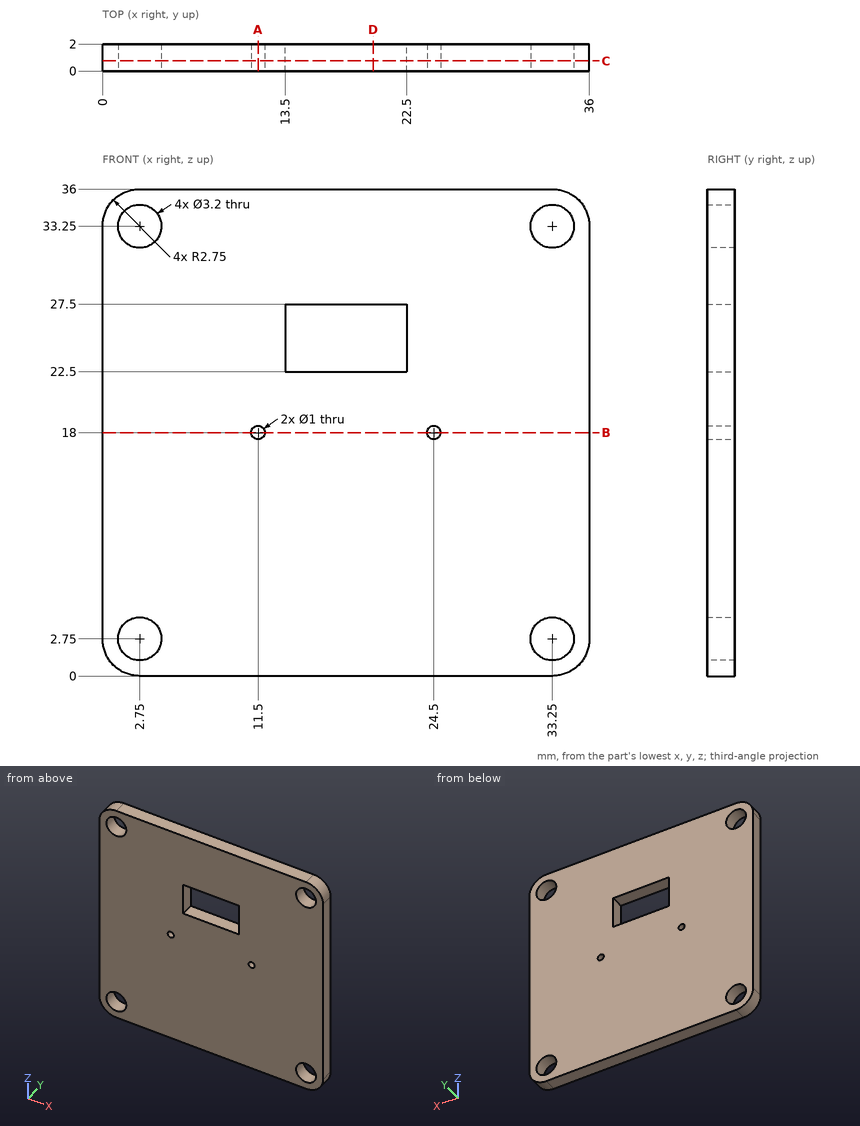
The drawing under review shows one solid part. Ordinate dimensions are in mm from its lowest x, y, z. Round coordinates to 2 decimals unless told otherwise and drop trailing zeros. Order: outer loops, then holes, each group sorted by start corner. A loop starts at its lowest first (then second) coordinate and runs counter-clockwise, first axis right, second up. Notation, with made-up numbers: (7.25, 78) -> (24.25, 78) arc R11 ccw to (24.25, 83) -> close; hole circle Ø8 at (48.5, 10.5). An arc over 180 degrees is marked (long way). Return JSON: item names as keys, results as strings.
1. For L1, parallel to X at y = 0.9, z = 33.25; L2, parallel to X at y = 1.15, z = 18; L3, parallel to Z at x = 16.5, y = 0.6, list the stretches that pass through material, from the lowest coordinate up. Write a range as [from, to].
Answer block:
{"L1": "x = [0, 1.15], [4.35, 31.65], [34.85, 36]", "L2": "x = [0, 11], [12, 24], [25, 36]", "L3": "z = [0, 22.5], [27.5, 36]"}
2. Take a section at B-B (z = 18). Write out the cut boundary in (x, y), then the cut area to 3 significant figures.
Answer block:
{"outline": "(0, 0) -> (11, 0) -> (11, 2) -> (0, 2) -> close; (12, 0) -> (24, 0) -> (24, 2) -> (12, 2) -> close; (25, 0) -> (36, 0) -> (36, 2) -> (25, 2) -> close", "area": "68.0 mm²"}
3. Take a section at A-A (x = 11.5). Write out the cut boundary in (y, z).
Answer block:
{"outline": "(0, 0) -> (2, 0) -> (2, 17.5) -> (0, 17.5) -> close; (0, 18.5) -> (2, 18.5) -> (2, 36) -> (0, 36) -> close"}
4. Insertion check: P1, Ø1.9, axis at x = 33.25, z = 2.75, coming from the -Y side. The pin has a flat end and moves straight along its axis. Give the tip position at first contact, or say it passes through.
Answer block:
{"P1": "passes through"}
5. Take a section at D-D (x = 20). Write out the cut boundary in (y, z).
Answer block:
{"outline": "(0, 0) -> (2, 0) -> (2, 22.5) -> (0, 22.5) -> close; (0, 27.5) -> (2, 27.5) -> (2, 36) -> (0, 36) -> close"}
6. Take a section at C-C (y = 0.75). Write out the cut boundary in (x, z).
Answer block:
{"outline": "(0, 2.75) arc R2.75 ccw to (2.75, 0) -> (33.25, 0) arc R2.75 ccw to (36, 2.75) -> (36, 33.25) arc R2.75 ccw to (33.25, 36) -> (2.75, 36) arc R2.75 ccw to (0, 33.25) -> close; hole circle Ø3.2 at (2.75, 2.75); hole circle Ø3.2 at (2.75, 33.25); hole circle Ø1 at (11.5, 18); hole (13.5, 22.5) -> (22.5, 22.5) -> (22.5, 27.5) -> (13.5, 27.5) -> close; hole circle Ø1 at (24.5, 18); hole circle Ø3.2 at (33.25, 2.75); hole circle Ø3.2 at (33.25, 33.25)"}
